Study the drawing (mm; zero at the part's minimum x, y, z) and answer. A direction names the side the tool comes from. Round coordinates to 2 decimals unless told otherwise and drop trailing zeros. Loops run counter-clockwise (first coordinate to the right, second up) from the corner with the lowest first, then second, coordinate; pieces in that order, holes last. Notation, with made-up numbers: (-17.75, 29.5) - (4.25, 29.5) arc R37 ccw to (4.25, 67.5) - close; hole circle Ø8 at (82, 66). An arc over 180 degrees is marked (long way). One line per item, written item: value.
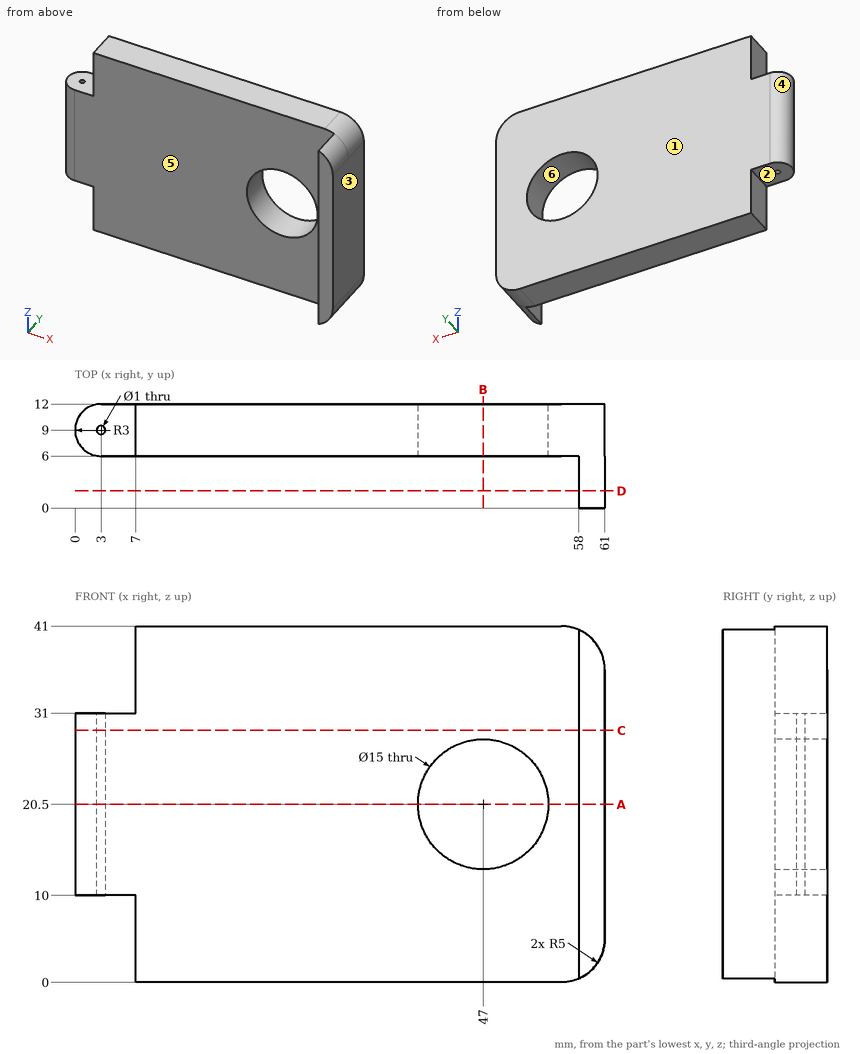
1) A cutting plane is placed at A-A on z = 20.5. Give the vertices of the cut face in (x, y).
Final values:
outline: (3, 6) - (39.5, 6) - (39.5, 12) - (3, 12) arc R3 ccw to start; (54.5, 6) - (58, 6) - (58, 0) - (61, 0) - (61, 12) - (54.5, 12) - close; hole circle Ø1 at (3, 9)
2) Consider L1, parallel to Y at x = 3, z = 16.75; L2, parallel to Y at x = 56, z = 16; L3, parallel to X at y = 2.5, z = 33.5. Determine where each line is inside the solid, lowest interval first.
Final values:
L1: 6 to 8.5, 9.5 to 12
L2: 6 to 12
L3: 58 to 61
3) A cutting plane is placed at C-C on z = 29. Give the vertices of the cut face in (x, y), and give its area (3 significant figures).
Final values:
outline: (3, 6) - (58, 6) - (58, 0) - (61, 0) - (61, 12) - (3, 12) arc R3 ccw to start; hole circle Ø1 at (3, 9)
area: 379 mm2
4) A cutting plane is placed at B-B on x = 47. Give the vertices of the cut face in (y, z).
Final values:
outline: (6, 0) - (12, 0) - (12, 13) - (6, 13) - close; (6, 28) - (12, 28) - (12, 41) - (6, 41) - close
5) For the marked faces 1 and 2, determine the directions among +Z, -Z, +X, -X, +Y, -Y from which every point of the face is accessible in a straight line to the end or side of a thin tool.
Final values:
face 1: +Z, -Z, +X, -X, +Y
face 2: -Z, -X, +Y, -Y
6) A cutting plane is placed at D-D on y = 2. Give the vertices of the cut face in (x, z).
Final values:
outline: (58, 0.42) arc R5 ccw to (61, 5) - (61, 36) arc R5 ccw to (58, 40.58) - close
7) For a pull along X with two mould halves and no side action, classify the marked faces 3, 4, 5 and 6 as released by +X, released by -X, zero draft, split by the parting line, or undercut.
Final values:
face 3: released by +X
face 4: released by -X
face 5: zero draft
face 6: undercut
8) Each of these flat-tipped pins is pushed along its axis until it touches: pin 1 Ø4 at (y, z) = (4.5, 33.5) entering from -X; pin 2 Ø1.8 at (y, z) = (2.5, 23) entering from -X; pin 3 Ø5 at (x, y) = (3, 9) entering from -Z. Where does it stop, or does it pass through?
Final values:
pin 1: x = 7
pin 2: x = 58
pin 3: z = 10
